Work out the finished part from the listing and answer in its coordinate system (mm). A direction names the side the tool comes from. Coordinates: 2 decimals unless noted, no trailing zeros. Loops run counter-clockwise (first coordinate to the right, second up) from the corner with the lowest first, then second, coordinate; pieces in that order, holes last. Notation, with made-up numbers: M 37,22.5 L 68,22.5 A20 ccw 68,37.5 Z; hole C 79,15.25 d8. An arc over 180 degrees is marked long. Write each question's results on one line, items separated by ' | '.
```python
from build123d import *
from build123d import SkipClean  # not in build123d's __all__

# Parameters (mm, degrees)
F0_R        = 42.6
F1_DEPTH    = 5
F2_DEPTH    = 15
F3_DEPTH    = 3
F4_START    = 5
F4_DEPTH    = 10
F5_T2_ANGLE = 88.4610047723
F5_T4_ANGLE = 87.6524613708
F5_T6_ANGLE = 88.4610047722
F5_T8_ANGLE = 87.9917435352


# Not quite as in the source:
# - a fillet or chamfer that OpenCascade refuses, or shapes differently, is made with other operations: its cross-section is extruded or revolved along the edge and cut away or added


with BuildPart() as f1:
    # F0 (on Top) → F1 (new body)
    with BuildSketch(Plane.XY):
        with BuildLine():
            Line((45, 0), (70, 0))
            ThreePointArc((70, 0), (69.9641265525, 2.2407578514), (69.8565429786, 4.4792190254))
            Line((69.8565429786, 4.4792190254), (44.7765183654, 4.4792190254))
            ThreePointArc((44.7765183654, 4.4792190254), (44.9440948648, 2.2423953219), (45, 0))
        make_face()
        with BuildLine():
            Line((44.7765183654, 4.4792190254), (69.8565429786, 4.4792190254))
            ThreePointArc((69.8565429786, 4.4792190254), (47.8876532533, 51.0565633968), (0, 70))
            Line((0, 70), (0, 61.6992585301))
            ThreePointArc((0, 61.6992585301), (3.6415999231, 60.1908584533), (5.15, 56.5492585301))
            ThreePointArc((5.15, 56.5492585301), (3.6415999231, 52.907658607), (0, 51.3992585301))
            Line((0, 51.3992585301), (0, 45))
            ThreePointArc((0, 45), (30.194661315, 33.3658871914), (44.7765183654, 4.4792190254))
        make_face()
        with BuildLine():
            Line((0, 61.6992585301), (0, 70))
            ThreePointArc((0, 70), (-1.9542396645, 69.972715735), (-3.9069559007, 69.8908842095))
            Line((-3.9069559007, 69.8908842095), (-3.9069559007, 59.9045820004))
            ThreePointArc((-3.9069559007, 59.9045820004), (-2.1497190663, 61.2291311711), (0, 61.6992585301))
        make_face()
        with BuildLine():
            Line((-3.9069559007, 59.9045820004), (-3.9069559007, 69.8908842095))
            ThreePointArc((-3.9069559007, 69.8908842095), (-49.2943701377, 49.699749222), (-69.8565429786, 4.4792190254))
            Line((-69.8565429786, 4.4792190254), (-44.7765183654, 4.4792190254))
            ThreePointArc((-44.7765183654, 4.4792190254), (-31.6159465637, 32.0223659788), (-3.9069559007, 44.8300757928))
            Line((-3.9069559007, 44.8300757928), (-3.9069559007, 53.1939350599))
            ThreePointArc((-3.9069559007, 53.1939350599), (-5.15, 56.5492585301), (-3.9069559007, 59.9045820004))
        make_face()
        with BuildLine():
            ThreePointArc((-69.8565429786, 4.4792190254), (-69.9641265525, 2.2407578514), (-70, 0))
            Line((-70, 0), (-45, 0))
            ThreePointArc((-45, 0), (-44.9440948648, 2.2423953219), (-44.7765183654, 4.4792190254))
            Line((-44.7765183654, 4.4792190254), (-69.8565429786, 4.4792190254))
        make_face()
        with BuildLine():
            ThreePointArc((-70, 0), (-49.4974746831, -49.4974746831), (0, -70))
            Line((0, -70), (0, -45))
            ThreePointArc((0, -45), (-31.8198051534, -31.8198051534), (-45, 0))
            Line((-45, 0), (-70, 0))
        make_face()
        with BuildLine():
            ThreePointArc((0, -70), (1.7470617825, -69.9781949976), (3.4930351455, -69.9127935751))
            Line((3.4930351455, -69.9127935751), (3.4930351455, -44.8642252298))
            ThreePointArc((3.4930351455, -44.8642252298), (1.7478364709, -44.9660434959), (0, -45))
            Line((0, -45), (0, -70))
        make_face()
        with BuildLine():
            ThreePointArc((3.4930351455, -69.9127935751), (50.7174154516, -48.2466969844), (70, 0))
            Line((70, 0), (45, 0))
            ThreePointArc((45, 0), (33.0317013, -30.5598872581), (3.4930351455, -44.8642252298))
            Line((3.4930351455, -44.8642252298), (3.4930351455, -69.9127935751))
        make_face()
        with BuildLine():
            Line((0, 51.3992585301), (0, 61.6992585301))
            ThreePointArc((0, 61.6992585301), (-2.1497190663, 61.2291311711), (-3.9069559007, 59.9045820004))
            Line((-3.9069559007, 59.9045820004), (-3.9069559007, 53.1939350599))
            ThreePointArc((-3.9069559007, 53.1939350599), (-2.1497190663, 51.8693858891), (0, 51.3992585301))
        make_face()
        with BuildLine():
            Line((-3.9069559007, 53.1939350599), (-3.9069559007, 59.9045820004))
            ThreePointArc((-3.9069559007, 59.9045820004), (-5.15, 56.5492585301), (-3.9069559007, 53.1939350599))
        make_face()
        with BuildLine():
            ThreePointArc((5.15, 56.5492585301), (3.6415999231, 60.1908584533), (0, 61.6992585301))
            Line((0, 61.6992585301), (0, 51.3992585301))
            ThreePointArc((0, 51.3992585301), (3.6415999231, 52.907658607), (5.15, 56.5492585301))
        make_face()
        with BuildLine():
            ThreePointArc((-3.9069559007, 44.8300757928), (-1.9553246946, 44.9574988777), (0, 45))
            Line((0, 45), (0, 51.3992585301))
            ThreePointArc((0, 51.3992585301), (-2.1497190663, 51.8693858891), (-3.9069559007, 53.1939350599))
            Line((-3.9069559007, 53.1939350599), (-3.9069559007, 44.8300757928))
        make_face()
        with BuildLine():
            ThreePointArc((3.4930351455, -44.8642252298), (33.0317013, -30.5598872581), (45, 0))
            ThreePointArc((45, 0), (44.9440948648, 2.2423953219), (44.7765183654, 4.4792190254))
            ThreePointArc((44.7765183654, 4.4792190254), (30.194661315, 33.3658871914), (0, 45))
            ThreePointArc((0, 45), (-1.9553246946, 44.9574988777), (-3.9069559007, 44.8300757928))
            ThreePointArc((-3.9069559007, 44.8300757928), (-31.6159465637, 32.0223659788), (-44.7765183654, 4.4792190254))
            ThreePointArc((-44.7765183654, 4.4792190254), (-44.9440948648, 2.2423953219), (-45, 0))
            ThreePointArc((-45, 0), (-31.8198051534, -31.8198051534), (0, -45))
            ThreePointArc((0, -45), (1.7478364709, -44.9660434959), (3.4930351455, -44.8642252298))
        make_face()
        Circle(F0_R, mode=Mode.SUBTRACT)
    extrude(amount=F1_DEPTH)

    # F0 (on Top) → F2 (join)
    with BuildSketch(Plane.XY):
        with BuildLine():
            ThreePointArc((3.4930351455, -44.8642252298), (33.0317013, -30.5598872581), (45, 0))
            ThreePointArc((45, 0), (44.9440948648, 2.2423953219), (44.7765183654, 4.4792190254))
            ThreePointArc((44.7765183654, 4.4792190254), (30.194661315, 33.3658871914), (0, 45))
            ThreePointArc((0, 45), (-1.9553246946, 44.9574988777), (-3.9069559007, 44.8300757928))
            ThreePointArc((-3.9069559007, 44.8300757928), (-31.6159465637, 32.0223659788), (-44.7765183654, 4.4792190254))
            ThreePointArc((-44.7765183654, 4.4792190254), (-44.9440948648, 2.2423953219), (-45, 0))
            ThreePointArc((-45, 0), (-31.8198051534, -31.8198051534), (0, -45))
            ThreePointArc((0, -45), (1.7478364709, -44.9660434959), (3.4930351455, -44.8642252298))
        make_face()
        Circle(F0_R, mode=Mode.SUBTRACT)
    extrude(amount=F2_DEPTH)

    # F0 (on Top) → F3 (cut)
    with BuildSketch(Plane.XY):
        with BuildLine():
            Line((0, 51.3992585301), (0, 61.6992585301))
            ThreePointArc((0, 61.6992585301), (-2.1497190663, 61.2291311711), (-3.9069559007, 59.9045820004))
            Line((-3.9069559007, 59.9045820004), (-3.9069559007, 53.1939350599))
            ThreePointArc((-3.9069559007, 53.1939350599), (-2.1497190663, 51.8693858891), (0, 51.3992585301))
        make_face()
        with BuildLine():
            ThreePointArc((5.15, 56.5492585301), (3.6415999231, 60.1908584533), (0, 61.6992585301))
            Line((0, 61.6992585301), (0, 51.3992585301))
            ThreePointArc((0, 51.3992585301), (3.6415999231, 52.907658607), (5.15, 56.5492585301))
        make_face()
        with BuildLine():
            Line((-3.9069559007, 53.1939350599), (-3.9069559007, 59.9045820004))
            ThreePointArc((-3.9069559007, 59.9045820004), (-5.15, 56.5492585301), (-3.9069559007, 53.1939350599))
        make_face()
    extrude(amount=F3_DEPTH, mode=Mode.SUBTRACT)

    # F0 (on Top) → F4 (join)
    with BuildSketch(Plane.XY.offset(F4_START)):
        with BuildLine():
            ThreePointArc((0, -70), (1.7470617825, -69.9781949976), (3.4930351455, -69.9127935751))
            Line((3.4930351455, -69.9127935751), (3.4930351455, -44.8642252298))
            ThreePointArc((3.4930351455, -44.8642252298), (1.7478364709, -44.9660434959), (0, -45))
            Line((0, -45), (0, -70))
        make_face()
        with BuildLine():
            ThreePointArc((-69.8565429786, 4.4792190254), (-69.9641265525, 2.2407578514), (-70, 0))
            Line((-70, 0), (-45, 0))
            ThreePointArc((-45, 0), (-44.9440948648, 2.2423953219), (-44.7765183654, 4.4792190254))
            Line((-44.7765183654, 4.4792190254), (-69.8565429786, 4.4792190254))
        make_face()
        with BuildLine():
            Line((45, 0), (70, 0))
            ThreePointArc((70, 0), (69.9641265525, 2.2407578514), (69.8565429786, 4.4792190254))
            Line((69.8565429786, 4.4792190254), (44.7765183654, 4.4792190254))
            ThreePointArc((44.7765183654, 4.4792190254), (44.9440948648, 2.2423953219), (45, 0))
        make_face()
        with BuildLine():
            Line((0, 51.3992585301), (0, 61.6992585301))
            ThreePointArc((0, 61.6992585301), (-2.1497190663, 61.2291311711), (-3.9069559007, 59.9045820004))
            Line((-3.9069559007, 59.9045820004), (-3.9069559007, 53.1939350599))
            ThreePointArc((-3.9069559007, 53.1939350599), (-2.1497190663, 51.8693858891), (0, 51.3992585301))
        make_face()
        with BuildLine():
            Line((0, 61.6992585301), (0, 70))
            ThreePointArc((0, 70), (-1.9542396645, 69.972715735), (-3.9069559007, 69.8908842095))
            Line((-3.9069559007, 69.8908842095), (-3.9069559007, 59.9045820004))
            ThreePointArc((-3.9069559007, 59.9045820004), (-2.1497190663, 61.2291311711), (0, 61.6992585301))
        make_face()
        with BuildLine():
            ThreePointArc((-3.9069559007, 44.8300757928), (-1.9553246946, 44.9574988777), (0, 45))
            Line((0, 45), (0, 51.3992585301))
            ThreePointArc((0, 51.3992585301), (-2.1497190663, 51.8693858891), (-3.9069559007, 53.1939350599))
            Line((-3.9069559007, 53.1939350599), (-3.9069559007, 44.8300757928))
        make_face()
    with SkipClean():  # cleaning this boolean's faces spoils the solid; the shape is the same uncleaned
        extrude(amount=F4_DEPTH)

    # F5: chamfer of 20 x 10 on 4 edges, made by hand

    # F5_s1 → F5_t2 (revolve, cut)
    with BuildSketch(Plane(origin=(0, 0, 0), x_dir=(0, 0, 1), z_dir=(-0.6742521694, -0.738501193, 0))):
        Polygon((5, -70), (15, -50), (15, -70), align=None)
    revolve(axis=Axis((0, 0, 15), (0, 0, 1)), revolution_arc=F5_T2_ANGLE, mode=Mode.SUBTRACT)

    # F5_s3 → F5_t4 (revolve, cut)
    with BuildSketch(Plane(origin=(0, 0, 0), x_dir=(0, 0, 1), z_dir=(-0.7385013236, 0.6742520264, 0))):
        Polygon((5, -70), (15, -50), (15, -70), align=None)
    revolve(axis=Axis((0, 0, 15), (0, 0, 1)), revolution_arc=F5_T4_ANGLE, mode=Mode.SUBTRACT)

    # F5_s5 → F5_t6 (revolve, cut)
    with BuildSketch(Plane(origin=(0, 0, 0), x_dir=(0, 0, 1), z_dir=(0.7201262035, 0.6938431026, 0))):
        Polygon((5, -70), (15, -50), (15, -70), align=None)
    revolve(axis=Axis((0, 0, 15), (0, 0, 1)), revolution_arc=F5_T6_ANGLE, mode=Mode.SUBTRACT)

    # F5_s7 → F5_t8 (revolve, cut)
    with BuildSketch(Plane(origin=(0, 0, 0), x_dir=(0, 0, 1), z_dir=(0.7385012727, -0.6742520821, 0))):
        Polygon((5, -70), (15, -50), (15, -70), align=None)
    revolve(axis=Axis((0, 0, 15), (0, 0, 1)), revolution_arc=F5_T8_ANGLE, mode=Mode.SUBTRACT)


solid = f1.part
```
1) Straight lines are drawn through the part: probe 1 along Z at (x, y) = (48, 37); probe 2 along Y at (x, z) = (50, 8); probe 3 along X at (y, z) = (-31, 4.75). For each, find the intervals that lie inside material, in ascending order. Write a range as [from, to].
Check result:
probe 1: [0, 5] | probe 2: [0, 4.48] | probe 3: [-62.76, -29.22], [29.22, 62.76]
2) Find section A-A, the plane y = -6. Give the vertices of the cut face in (x, z), and give its area (3 significant figures).
Check result:
outline: M -69.74,0 L -42.18,0 L -42.18,15 L -44.6,15 L -44.6,5 L -69.74,5 Z; M 42.18,0 L 69.74,0 L 69.74,5 L 44.6,5 L 44.6,15 L 42.18,15 Z | area: 324 mm^2
3) Which of the six approach directions +Z, -Z, +X, -X, +Y, -Y give full straight-line access (tool end or side, diameter ignored) to faces 4 (the face through (0, 55, 9)), 5 (the face through (-37, 38, 5)), 6 (the face through (36, -34, 5)), 7 (the face through (-32.168, -31.468, 9.93))?
Check result:
face 4: +Z, +X, +Y | face 5: +Z, -X, +Y | face 6: +Z, +X, -Y | face 7: +Z, -X, -Y
4) Find section B-B, the plane x = -31. Give the vertices of the cut face in (y, z).
Check result:
outline: M -62.76,0 L -29.22,0 L -29.22,15 L -32.62,15 L -32.62,5 L -62.76,5 Z; M 29.22,0 L 62.76,0 L 62.76,5 L 32.62,5 L 32.62,15 L 29.22,15 Z
5) Find section C-C, the plane z = 8. Give the vertices of the cut face in (x, y), and give its area (3 significant figures).
Check result:
outline: M -64,0 L -45,0 A45 ccw 0,-45 L 0,-64 A64 ccw 3.49,-63.9 L 3.49,-44.86 A45 ccw 45,0 L 64,0 A64 ccw 63.84,4.48 L 44.78,4.48 A45 ccw 0,45 L 0,64 A64 ccw -3.91,63.88 L -3.91,44.83 A45 ccw -44.78,4.48 L -63.84,4.48 A64 ccw Z; hole C 0,0 d85.2 | area: 972 mm^2
6) For a pull along Y with two mould halves and no side action, classify faces 1 (the face through (32.711, -30.903, 9.93)), 2 (the face through (-35, -35, 5)), 3 (the face through (0, 57, 3)) as released by +Y, released by -Y, zero draft, split by the parting line, or undercut.
Check result:
face 1: released by -Y | face 2: zero draft | face 3: undercut
7) Given pin 1 Ø2 at (x, z) = (-39.5, 6.5) entering from +Y; pin 2 Ø5 at (y, z) = (-55.5, 9.5) entering from -X; pin 3 Ø5 at (y, z) = (-61, 11) entering from +X, each flat-ended and moving along its own axis, determine where each tip first touches the part or whether it passes through.
Check result:
pin 1: y = 23.3 | pin 2: x = 0 | pin 3: x = 3.49
